```python
from build123d import *

# Parameters (mm, degrees)
SKETCH1_W           = 84
SKETCH1_H           = 137
BOSS_EXTRUDE1_DEPTH = 3
BOSS_EXTRUDE2_DEPTH = 1
FILLET1_R           = 5
SKETCH4_R           = 2.5
CUT_EXTRUDE1_DEPTH  = 5
SKETCH5_R           = 3.5
CUT_EXTRUDE2_DEPTH  = 3.5
SKETCH6_W           = 60
SKETCH6_H           = 113
CUT_EXTRUDE3_DEPTH  = 4
SKETCH7_W           = 79.5
SKETCH7_H           = 113
CUT_EXTRUDE4_DEPTH  = 1
CHAMFER1_SIZE       = 1.75


with BuildPart() as part:
    # Sketch1 → Boss-Extrude1 (new body)
    with BuildSketch(Plane(origin=(0, 0, 0), x_dir=(1, 0, 0), z_dir=(0, 1, 0))):
        with Locations((42, 68.5)):
            Rectangle(SKETCH1_W, SKETCH1_H)
    extrude(amount=BOSS_EXTRUDE1_DEPTH)

    # Sketch3 → Boss-Extrude2 (add)
    with BuildSketch(Plane(origin=(0, 3, 0), x_dir=(1, 0, 0), z_dir=(0, 1, 0))):
        with BuildLine():
            Line((81.75, 125), (72, 125))
            Line((72, 125), (72, 134.75))
            Line((72, 134.75), (79, 134.75))
            ThreePointArc((79, 134.75), (80.944543648, 133.944543648), (81.75, 132))
            Line((81.75, 132), (81.75, 125))
        make_face()
        with BuildLine():
            Line((12, 2.25), (12, 12))
            Line((12, 12), (2.25, 12))
            Line((2.25, 12), (2.25, 5))
            ThreePointArc((2.25, 5), (3.055456352, 3.055456352), (5, 2.25))
            Line((5, 2.25), (12, 2.25))
        make_face()
    extrude(amount=BOSS_EXTRUDE2_DEPTH)

    # Fillet1
    fillet1_edges = [part.edges().sort_by_distance(p)[0] for p in [
        (0, 1.5, -137),
        (84, 1.5, -137),
        (84, 1.5, 0),
        (0, 1.5, 0),
    ]]
    fillet(fillet1_edges, radius=FILLET1_R)

    # Sketch4 → Cut-Extrude1 (cut, through all)
    with BuildSketch(Plane(origin=(0, 4, 0), x_dir=(1, 0, 0), z_dir=(0, 1, 0))):
        with Locations((7, 7)):
            Circle(SKETCH4_R)
        with Locations((77, 130)):
            Circle(SKETCH4_R)
    extrude(amount=-CUT_EXTRUDE1_DEPTH, mode=Mode.SUBTRACT)

    # Sketch5 → Cut-Extrude2 (cut, through all)
    with BuildSketch(Plane(origin=(0, 2.5, 0), x_dir=(1, 0, 0), z_dir=(0, 1, 0))):
        with Locations((7, 7)):
            Circle(SKETCH5_R)
        with Locations((77, 130)):
            Circle(SKETCH5_R)
    extrude(amount=-CUT_EXTRUDE2_DEPTH, mode=Mode.SUBTRACT)

    # Sketch6 → Cut-Extrude3 (cut, through all)
    with BuildSketch(Plane(origin=(0, 3, 0), x_dir=(1, 0, 0), z_dir=(0, 1, 0))):
        with Locations((42, 68.5)):
            Rectangle(SKETCH6_W, SKETCH6_H)
    extrude(amount=-CUT_EXTRUDE3_DEPTH, mode=Mode.SUBTRACT)

    # Sketch7 → Cut-Extrude4 (cut)
    with BuildSketch(Plane(origin=(0, 3, 0), x_dir=(1, 0, 0), z_dir=(0, 1, 0))):
        with Locations((42, 68.5)):
            Rectangle(SKETCH7_W, SKETCH7_H)
    extrude(amount=-CUT_EXTRUDE4_DEPTH, mode=Mode.SUBTRACT)

    # Chamfer1
    chamfer1_edges = [part.edges().sort_by_distance(p)[0] for p in [
        (84, 0, -68.5),
        (0, 0, -68.5),
        (42, 0, -137),
        (42, 0, 0),
        (82.535533906, 0, -135.535533906),
        (1.464466094, 0, -135.535533906),
        (1.464466094, 0, -1.464466094),
        (82.535533906, 0, -1.464466094),
    ]]
    chamfer(chamfer1_edges, length=CHAMFER1_SIZE)


solid = part.part
```
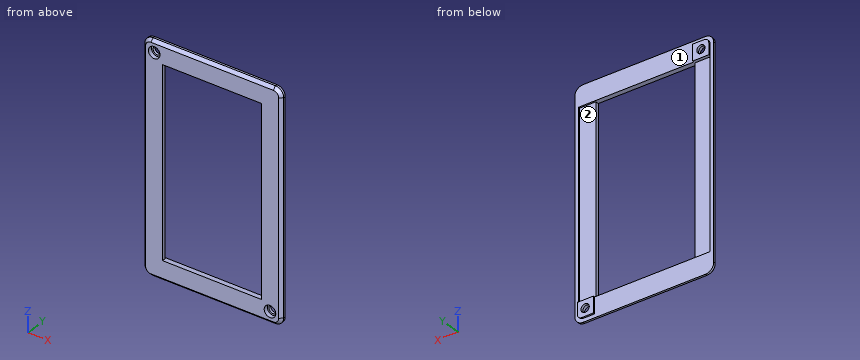
Here's how the part is built. I have some questions about the finished solid (model axes, mm). Face numbers are marked on the shaded views. Coordinates: 2 decimals unless noted, no trailing zeros. Order: outer loops, then holes, each group sorted by start corner. A loop starts at its lowest first (then second) coordinate and runs counter-clockwise, first axis right, second up. Notation, with made-up numbers: (87.25, -1) - (92.25, -1) arc R27 ccw to (92.25, 20) - close; hole circle Ø7 at (87, 42.5). An arc over 180 degrees is marked (long way). One line per question, with ' | ' between items.
(1) Suppose I cut it at A-A on y = 0.95. List the corners of the cut face in (x, z) for me, and give its area (3 significant figures).
Report:
outline: (0.8, -132) arc R4.2 ccw to (5, -136.2) - (79, -136.2) arc R4.2 ccw to (83.2, -132) - (83.2, -5) arc R4.2 ccw to (79, -0.8) - (5, -0.8) arc R4.2 ccw to (0.8, -5) - close; hole circle Ø7 at (7, -7); hole (12, -125) - (72, -125) - (72, -12) - (12, -12) - close; hole circle Ø7 at (77, -130) | area: 4,280 mm2
(2) Suppose I cut it at C-C on z = -47. List the corners of the cut face in (x, y) for me.
Report:
outline: (0, 1.75) - (1.75, 0) - (12, 0) - (12, 2) - (2.25, 2) - (2.25, 3) - (0, 3) - close; (72, 0) - (82.25, 0) - (84, 1.75) - (84, 3) - (81.75, 3) - (81.75, 2) - (72, 2) - close
(3) If we mould it in two halves opening along X, with no side actions, what happens to the marked faces 1 and 2? For each: pulls with the +X half, pulls with the -X half, needs draft (parallel to the pull), parting line crosses it, or undercut.
Report:
face 1: needs draft | face 2: undercut
(4) Suppose I cut it at D-D on x = 27.5. List the corners of the cut face in (y, z) for me.
Report:
outline: (0, -135.25) - (1.75, -137) - (3, -137) - (3, -125) - (0, -125) - close; (0, -12) - (3, -12) - (3, 0) - (1.75, 0) - (0, -1.75) - close
(5) If I drill on L1, parallel to Z at x = 77, y = 2.8; L2, parallel to X at y = 3.2, z = -7; L3, parallel to Z at x = 77, y = 3.65, over which ranges is the centre line in solid material (lowest first)?
Report:
L1: z = -137 to -132.5, -127.5 to -125, -12 to 0 | L2: x = 2.25 to 4.5, 9.5 to 12 | L3: z = -134.75 to -132.5, -127.5 to -125
(6) Will these pins go through, and if not, where does the flat tip stop? pin 1 (6 mm diameter, centred on x = 67.5, z = -43, fed in from -Y); pin 2 (8 mm diameter, centred on x = 7, z = -54, fed in from +Y); pin 3 (0.6 mm diameter, centred on y = 1, z = -62.5, fed in from +X).
Report:
pin 1: passes through | pin 2: stops at y = 2 | pin 3: stops at x = 83.55
(7) Suppose I cut it at B-B on x = 77. List the corners of the cut face in (y, z) for me.
Report:
outline: (0, -135.25) - (1.75, -137) - (3, -137) - (3, -134.75) - (4, -134.75) - (4, -132.5) - (2.5, -132.5) - (2.5, -133.5) - (0, -133.5) - close; (0, -126.5) - (2.5, -126.5) - (2.5, -127.5) - (4, -127.5) - (4, -125) - (2, -125) - (2, -12) - (3, -12) - (3, 0) - (1.75, 0) - (0, -1.75) - close
